from build123d import *

# Parameters (mm, degrees)
F1_DEPTH = 8
F2_DEPTH = 3
F3_W     = 10
F3_H     = 10
F4_DEPTH = 8


with BuildPart() as f1:
    # F0 (on Top) → F1 (new body)
    with BuildSketch(Plane.XY):
        with BuildLine():
            ThreePointArc((0, 2.85), (-2.0152543264, -2.0152543264), (2.85, 0))
            ThreePointArc((2.85, 0), (2.0152543264, 2.0152543264), (0, 2.85))
        make_face()
        with BuildLine():
            ThreePointArc((-1.8812210579, -1.4083704525), (-2.1014483771, 1.0518624997), (0, 2.35))
            ThreePointArc((0, 2.35), (1.6617009358, 1.6617009358), (2.35, 0))
            ThreePointArc((2.35, 0), (2.2297275042, -0.7421692913), (1.8812210579, -1.4083704525))
            ThreePointArc((1.8812210579, -1.4083704525), (0, -2.35), (-1.8812210579, -1.4083704525))
        make_face(mode=Mode.SUBTRACT)
        with BuildLine():
            ThreePointArc((2.35, 0), (1.6617009358, 1.6617009358), (0, 2.35))
            Line((0, 2.35), (0, 1.85))
            Line((0, 1.85), (1.5588457268, -0.85))
            Line((1.5588457268, -0.85), (1.8812210579, -1.4083704525))
            ThreePointArc((1.8812210579, -1.4083704525), (2.2297275042, -0.7421692913), (2.35, 0))
        make_face()
        with BuildLine():
            Line((0, 1.85), (0, 2.35))
            ThreePointArc((0, 2.35), (-2.1014483771, 1.0518624997), (-1.8812210579, -1.4083704525))
            Line((-1.8812210579, -1.4083704525), (-1.5588457268, -0.85))
            Line((-1.5588457268, -0.85), (0, 1.85))
        make_face()
    extrude(amount=F1_DEPTH)

    # F0 (on Top) → F2 (join)
    with BuildSketch(Plane.XY):
        with BuildLine():
            Line((-1.5588457268, -0.85), (-1.8812210579, -1.4083704525))
            ThreePointArc((-1.8812210579, -1.4083704525), (0, -2.35), (1.8812210579, -1.4083704525))
            Line((1.8812210579, -1.4083704525), (1.5588457268, -0.85))
            Line((1.5588457268, -0.85), (0, 1.85))
            Line((0, 1.85), (-1.5588457268, -0.85))
        make_face()
    extrude(amount=F2_DEPTH)

    # F3 (on Top) → F4 (join)
    with BuildSketch(Plane.XY):
        Rectangle(F3_W, F3_H)
    extrude(amount=-F4_DEPTH)


solid = f1.part
Design review of the part built by this model. Coordinates are the model's own, in mm. A direction names the side the tool comes from. Round coordinates to 2 decimals unless told otherwise and drop trailing zeros. Order: outer loops, then holes, each group sorted by start corner. A loop starts at its lowest first (then second) coordinate and runs counter-clockwise, first axis right, second up.
1) Consider section C-C (y = 2.25). State the section outline as (x, z) points, plus the area to 3 significant figures.
The answers:
outline: (-5, -8) - (5, -8) - (5, 0) - (1.75, 0) - (1.75, 8) - (-1.75, 8) - (-1.75, 0) - (-5, 0) - close
area: 108 mm2
2) Draft analysis for pull direction X (two halves, no side actions). For faces 3 (the flat face through (0, 0, -8)), 4 (the flat face through (5, 0, -4)), 5 (the cylindrical face through (0.03, -2.35, 5.46)), state which applies: released by +X, released by -X, zero draft, split by the parting line, or undercut.
The answers:
face 3: zero draft
face 4: released by +X
face 5: undercut
3) For L1, parallel to Z at x = -4.5, y = 0.5; L2, parallel to X at y = -0.75, z = 3.25; L3, parallel to Y at x = -0.5, z = 5, list the stretches that pass through material, from the lowest coordinate up.
The answers:
L1: z = -8 to 0
L2: x = -2.75 to -1.5, 1.5 to 2.75
L3: y = -2.81 to -2.3, 0.98 to 2.81
4) Consider section B-B (x = 2.5). State the section outline as (y, z) points, plus the area to 3 significant figures.
The answers:
outline: (-5, -8) - (5, -8) - (5, 0) - (1.37, 0) - (1.37, 8) - (-1.37, 8) - (-1.37, 0) - (-5, 0) - close
area: 102 mm2
5) Consider section D-D (z = 0.25). State the section outline as (x, y) points.
The answers:
outline: circle Ø5.7 at (0, 0)
6) Consider section A-A (z = 6). State the section outline as (x, y) points.
The answers:
outline: circle Ø5.7 at (0, 0); hole (-1.88, -1.41) arc R2.35 ccw to (1.88, -1.41) - (0, 1.85) - close
7) Machinability: for faces 1 (the flat face through (2.2, 2.3, 0)), 2 (the flat face through (-5, 0, -4)), which of the approach directions +Z, -Z, +X, -X, +Y, -Y give a long, thin tool a straight path to every point of the face, cutting with its end or side? Answer none if there is none.
The answers:
face 1: +Z
face 2: +Z, -Z, -X, +Y, -Y
8) Clearance check with flat-ended pins moving along their axes: pin 1 Ø3 at (y, z) = (3, 5) entering from -X; pin 2 Ø3 at (x, z) = (-3.5, 6.5) entering from +Y. State where each tip first meets the part, or that it passes through.
The answers:
pin 1: stops at x = -2.42
pin 2: stops at y = 2.03
